```python
from build123d import *

# Parameters (mm, degrees)
SKETCH_1_R          = 1.75
SKETCH_1_R_2        = 1.3
EXTRUDE_1_DEPTH     = 2
SKETCH_2_W          = 20.4
SKETCH_2_H          = 41
CUT_EXTRUDE_1_DEPTH = 238.073828163
SKETCH_3_W          = 6.060289077
SKETCH_3_H          = 20
EXTRUDE_2_DEPTH     = 2
FILLET_3_R          = 5
FILLET_4_R          = 5
FILLET_5_R          = 5
FILLET_6_R          = 5


with BuildPart() as part:
    # 草图1 → 凸台-拉伸1 (new body)
    with BuildSketch(Plane.XY):
        with BuildLine():
            Line((7.8, 0), (202.2, 0))
            ThreePointArc((202.2, 0), (204.321320344, -0.878679656), (205.2, -3))
            Line((205.2, -3), (205.2, -20))
            Line((205.2, -20), (207, -20))
            ThreePointArc((207, -20), (209.121320344, -19.121320344), (210, -17))
            Line((210, -17), (210, 0))
            Line((210, 0), (210, 90))
            Line((210, 90), (210, 107))
            ThreePointArc((210, 107), (209.121320344, 109.121320344), (207, 110))
            Line((207, 110), (205.2, 110))
            Line((205.2, 110), (205.2, 93))
            ThreePointArc((205.2, 93), (204.321320344, 90.878679656), (202.2, 90))
            Line((202.2, 90), (7.8, 90))
            ThreePointArc((7.8, 90), (5.678679656, 90.878679656), (4.8, 93))
            Line((4.8, 93), (4.8, 110))
            Line((4.8, 110), (3, 110))
            ThreePointArc((3, 110), (0.878679656, 109.121320344), (0, 107))
            Line((0, 107), (0, 90))
            Line((0, 90), (0, 0))
            Line((0, 0), (0, -17))
            ThreePointArc((0, -17), (0.878679656, -19.121320344), (3, -20))
            Line((3, -20), (4.8, -20))
            Line((4.8, -20), (4.8, -3))
            ThreePointArc((4.8, -3), (5.678679656, -0.878679656), (7.8, 0))
        make_face()
        with Locations((2.5, 53)):
            Circle(SKETCH_1_R, mode=Mode.SUBTRACT)
        with Locations(Location((17.5, 53, 0), (0, 0, 180))):
            Circle(SKETCH_1_R, mode=Mode.SUBTRACT)
        with Locations((17.5, 37)):
            Circle(SKETCH_1_R, mode=Mode.SUBTRACT)
        with Locations(Location((2.5, 37, 0), (0, 0, 180))):
            Circle(SKETCH_1_R, mode=Mode.SUBTRACT)
        with Locations((207.5, 37)):
            Circle(SKETCH_1_R, mode=Mode.SUBTRACT)
        with Locations(Location((192.5, 37, 0), (0, 0, 180))):
            Circle(SKETCH_1_R, mode=Mode.SUBTRACT)
        with Locations((192.5, 53)):
            Circle(SKETCH_1_R, mode=Mode.SUBTRACT)
        with Locations(Location((207.5, 53, 0), (0, 0, 180))):
            Circle(SKETCH_1_R, mode=Mode.SUBTRACT)
        with Locations((28, 83)):
            Circle(SKETCH_1_R_2, mode=Mode.SUBTRACT)
        with Locations(Location((182, 83, 0), (0, 0, 180))):
            Circle(SKETCH_1_R_2, mode=Mode.SUBTRACT)
        with Locations((182, 7)):
            Circle(SKETCH_1_R_2, mode=Mode.SUBTRACT)
        with Locations(Location((28, 7, 0), (0, 0, 180))):
            Circle(SKETCH_1_R_2, mode=Mode.SUBTRACT)
        with BuildLine():
            Line((22, 71.710263165), (22, 53))
            ThreePointArc((22, 53), (22.878679656, 50.878679656), (25, 50))
            Line((25, 50), (40.583105292, 50))
            ThreePointArc((40.583105292, 50), (43.299697276, 51.727157515), (42.888301086, 54.919914673))
            Line((42.888301086, 54.919914673), (27.305195794, 73.630177837))
            ThreePointArc((27.305195794, 73.630177837), (23.979114939, 74.531219331), (22, 71.710263165))
        make_face(mode=Mode.SUBTRACT)
        with BuildLine():
            Line((39.111698914, 75.080085327), (57.767217115, 52.680849201))
            ThreePointArc((57.767217115, 52.680849201), (60.025200787, 51.601135394), (62.316045524, 52.60925372))
            Line((62.316045524, 52.60925372), (82.19822493, 75.008489847))
            ThreePointArc((82.19822493, 75.008489847), (82.690879074, 78.229932832), (79.954592315, 80))
            Line((79.954592315, 80), (41.416894708, 80))
            ThreePointArc((41.416894708, 80), (38.700302724, 78.272842485), (39.111698914, 75.080085327))
        make_face(mode=Mode.SUBTRACT)
        with BuildLine():
            Line((100, 72.101020514), (100, 53))
            ThreePointArc((100, 53), (99.121320344, 50.878679656), (97, 50))
            Line((97, 50), (80.045407685, 50))
            ThreePointArc((80.045407685, 50), (77.309120926, 51.770067168), (77.80177507, 54.991510153))
            Line((77.80177507, 54.991510153), (94.756367385, 74.092530668))
            ThreePointArc((94.756367385, 74.092530668), (98.065153077, 74.905561283), (100, 72.101020514))
        make_face(mode=Mode.SUBTRACT)
        with BuildLine():
            Line((113, 50), (129.954592315, 50))
            ThreePointArc((129.954592315, 50), (132.690879074, 51.770067168), (132.19822493, 54.991510153))
            Line((132.19822493, 54.991510153), (115.243632615, 74.092530668))
            ThreePointArc((115.243632615, 74.092530668), (111.934846923, 74.905561283), (110, 72.101020514))
            Line((110, 72.101020514), (110, 53))
            ThreePointArc((110, 53), (110.878679656, 50.878679656), (113, 50))
        make_face(mode=Mode.SUBTRACT)
        with BuildLine():
            Line((147.683954476, 52.60925372), (127.80177507, 75.008489847))
            ThreePointArc((127.80177507, 75.008489847), (127.309120926, 78.229932832), (130.045407685, 80))
            Line((130.045407685, 80), (168.583105292, 80))
            ThreePointArc((168.583105292, 80), (171.299697276, 78.272842485), (170.888301086, 75.080085327))
            Line((170.888301086, 75.080085327), (152.232782885, 52.680849201))
            ThreePointArc((152.232782885, 52.680849201), (149.974799213, 51.601135394), (147.683954476, 52.60925372))
        make_face(mode=Mode.SUBTRACT)
        with BuildLine():
            Line((167.111698914, 54.919914673), (182.694804206, 73.630177837))
            ThreePointArc((182.694804206, 73.630177837), (186.020885061, 74.531219331), (188, 71.710263165))
            Line((188, 71.710263165), (188, 53))
            ThreePointArc((188, 53), (187.121320344, 50.878679656), (185, 50))
            Line((185, 50), (169.416894708, 50))
            ThreePointArc((169.416894708, 50), (166.700302724, 51.727157515), (167.111698914, 54.919914673))
        make_face(mode=Mode.SUBTRACT)
        with BuildLine():
            Line((185, 40), (169.416894708, 40))
            ThreePointArc((169.416894708, 40), (166.700302724, 38.272842485), (167.111698914, 35.080085327))
            Line((167.111698914, 35.080085327), (182.694804206, 16.369822163))
            ThreePointArc((182.694804206, 16.369822163), (186.020885061, 15.468780669), (188, 18.289736835))
            Line((188, 18.289736835), (188, 37))
            ThreePointArc((188, 37), (187.121320344, 39.121320344), (185, 40))
        make_face(mode=Mode.SUBTRACT)
        with BuildLine():
            Line((170.888301086, 14.919914673), (152.232782885, 37.319150799))
            ThreePointArc((152.232782885, 37.319150799), (149.974799213, 38.398864606), (147.683954476, 37.39074628))
            Line((147.683954476, 37.39074628), (127.80177507, 14.991510153))
            ThreePointArc((127.80177507, 14.991510153), (127.309120926, 11.770067168), (130.045407685, 10))
            Line((130.045407685, 10), (168.583105292, 10))
            ThreePointArc((168.583105292, 10), (171.299697276, 11.727157515), (170.888301086, 14.919914673))
        make_face(mode=Mode.SUBTRACT)
        with BuildLine():
            Line((113, 40), (129.954592315, 40))
            ThreePointArc((129.954592315, 40), (132.690879074, 38.229932832), (132.19822493, 35.008489847))
            Line((132.19822493, 35.008489847), (115.243632615, 15.907469332))
            ThreePointArc((115.243632615, 15.907469332), (111.934846923, 15.094438717), (110, 17.898979486))
            Line((110, 17.898979486), (110, 37))
            ThreePointArc((110, 37), (110.878679656, 39.121320344), (113, 40))
        make_face(mode=Mode.SUBTRACT)
        with BuildLine():
            Line((97, 40), (80.045407685, 40))
            ThreePointArc((80.045407685, 40), (77.309120926, 38.229932832), (77.80177507, 35.008489847))
            Line((77.80177507, 35.008489847), (94.756367385, 15.907469332))
            ThreePointArc((94.756367385, 15.907469332), (98.065153077, 15.094438717), (100, 17.898979486))
            Line((100, 17.898979486), (100, 37))
            ThreePointArc((100, 37), (99.121320344, 39.121320344), (97, 40))
        make_face(mode=Mode.SUBTRACT)
        with BuildLine():
            Line((62.316045524, 37.39074628), (82.19822493, 14.991510153))
            ThreePointArc((82.19822493, 14.991510153), (82.690879074, 11.770067168), (79.954592315, 10))
            Line((79.954592315, 10), (41.416894708, 10))
            ThreePointArc((41.416894708, 10), (38.700302724, 11.727157515), (39.111698914, 14.919914673))
            Line((39.111698914, 14.919914673), (57.767217115, 37.319150799))
            ThreePointArc((57.767217115, 37.319150799), (60.025200787, 38.398864606), (62.316045524, 37.39074628))
        make_face(mode=Mode.SUBTRACT)
        with BuildLine():
            Line((42.888301086, 35.080085327), (27.305195794, 16.369822163))
            ThreePointArc((27.305195794, 16.369822163), (23.979114939, 15.468780669), (22, 18.289736835))
            Line((22, 18.289736835), (22, 37))
            ThreePointArc((22, 37), (22.878679656, 39.121320344), (25, 40))
            Line((25, 40), (40.583105292, 40))
            ThreePointArc((40.583105292, 40), (43.299697276, 38.272842485), (42.888301086, 35.080085327))
        make_face(mode=Mode.SUBTRACT)
    extrude(amount=EXTRUDE_1_DEPTH)

    # 草图2 → 切除-拉伸1 (cut, through all)
    with BuildSketch(Plane.XY.offset(2)):
        with Locations((10.2, 45)):
            Rectangle(SKETCH_2_W, SKETCH_2_H)
        with Locations((199.8, 45)):
            Rectangle(SKETCH_2_W, SKETCH_2_H)
    extrude(amount=-CUT_EXTRUDE_1_DEPTH, mode=Mode.SUBTRACT)

    # 草图3 → 凸台-拉伸2 (add)
    with BuildSketch(Plane.XY.offset(2)):
        with Locations((7.830144539, 100)):
            Rectangle(SKETCH_3_W, SKETCH_3_H)
        with Locations((202.169855462, 100)):
            Rectangle(SKETCH_3_W, SKETCH_3_H)
        with Locations((202.169855462, -10)):
            Rectangle(SKETCH_3_W, SKETCH_3_H)
        with Locations((7.830144539, -10)):
            Rectangle(SKETCH_3_W, SKETCH_3_H)
    extrude(amount=-EXTRUDE_2_DEPTH)

    # 圆角3
    fillet_3_edges = [part.edges().sort_by_distance(p)[0] for p in [
        (10.860289077, 0, 1),
    ]]
    fillet(fillet_3_edges, radius=FILLET_3_R)

    # 圆角4
    fillet_4_edges = [part.edges().sort_by_distance(p)[0] for p in [
        (199.139710923, 0, 1),
    ]]
    fillet(fillet_4_edges, radius=FILLET_4_R)

    # 圆角5
    fillet_5_edges = [part.edges().sort_by_distance(p)[0] for p in [
        (199.139710923, 90, 1),
    ]]
    fillet(fillet_5_edges, radius=FILLET_5_R)

    # 圆角6
    fillet_6_edges = [part.edges().sort_by_distance(p)[0] for p in [
        (10.860289077, 90, 1),
    ]]
    fillet(fillet_6_edges, radius=FILLET_6_R)


solid = part.part
```
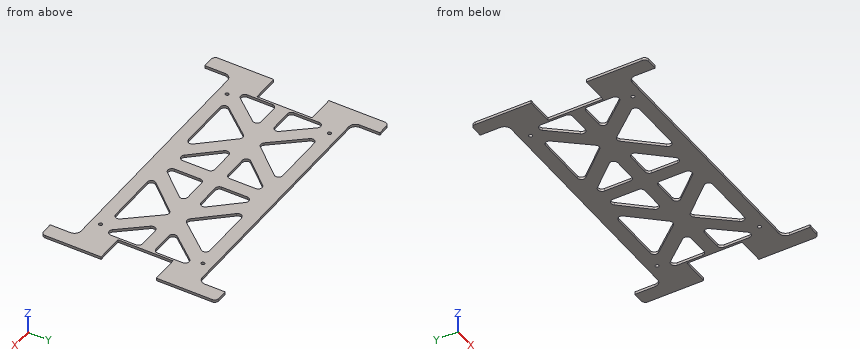
Check sheet for the modelled part. Datum: model origin and axes. Units: mm. Round coordinates to 2 decimals unless told otherwise and drop trailing zeros. Order: outer loops, then holes, each group sorted by start corner. A loop starts at its lowest first (then second) coordinate and runs counter-clockwise, first axis right, second up. Notation, with made-up numbers: (10, 46) - (23, 46) arc R15 cw to (23, 74) - close; hole circle Ø5 at (-19, 48.5). An arc over 180 degrees is marked (long way). Write item = value, one per line.
Q1. Section check B-B (x = 144.5). Record the boundary of the cut face in (y, z).
Computed:
outline = (0, 0) - (10, 0) - (10, 2) - (0, 2) - close; (33.8, 0) - (56.2, 0) - (56.2, 2) - (33.8, 2) - close; (80, 0) - (90, 0) - (90, 2) - (80, 2) - close
Q2. Go/stop test with flat-tipped pins: pin 1 (0.6 mm diameter, centred on x = 179, z = 1.5, fed in from +Y); pin 2 (4 mm diameter, centred on x = 129.5, y = 92.5, fed in from -Z); pin 3 (1 mm diameter, centred on y = 61.5, z = 1.5, fed in from +X); pin 4 (1 mm diameter, centred on x = 64.5, z = 1.5, fed in from -Y). Record where each tip stops, or that it passes through.
Computed:
pin_1 = 90
pin_2 = through
pin_3 = 189.6
pin_4 = 0
Q3. Section check C-C (z = 1). State how many separate pieces and enclosed holes the cut face has, and give its area (3 significant figures).
Computed:
separate_pieces = 1
enclosed_holes = 16
area = 12,200 mm^2
Q4. Thickness scan on line 1 along X through (y, z) = (83, 1.2); line 2 along Y through (x, z) = (10, 1.9); line 3 along X through (y, z) = (-10.5, 1). Record the ranges inside material, lowest first.
Computed:
line_1 = 0 to 26.7, 29.3 to 180.7, 183.3 to 210
line_2 = -20 to 24.5, 65.5 to 110
line_3 = 0 to 10.86, 199.14 to 210
Q5. Section check A-A (y = 92.5). Record the boundary of the cut face in (x, z), and give its area (3 significant figures).
Computed:
outline = (0, 0) - (11.53, 0) - (11.53, 2) - (0, 2) - close; (198.47, 0) - (210, 0) - (210, 2) - (198.47, 2) - close
area = 46.1 mm^2
Q6. Section check D-D (x = 48). Record the boundary of the cut face in (y, z), and give its area (3 significant figures).
Computed:
outline = (0, 0) - (10, 0) - (10, 2) - (0, 2) - close; (25.59, 0) - (64.41, 0) - (64.41, 2) - (25.59, 2) - close; (80, 0) - (90, 0) - (90, 2) - (80, 2) - close
area = 118 mm^2
